Check sheet for the modelled part. Datum: model origin and axes. Units: mm. Face numbers are marked on the shaded views. A direction names the side the tool comes from. Coordinates: 2 decimals unless noted, no trailing zeros. Loops run counter-clockwise (first coordinate to the right, second up) from the corner with the lowest first, then second, coordinate; pieces in that order, holes last. Notation, with made-up numbers: M 16.5,-8 L 42.5,-8 A13 ccw 42.5,12 Z; hole C 14,50 d11. An arc over 180 degrees is marked long. Use CSV: the item, a comma, the result in double quotes. Start each with the question number.
(1) Section check B-B on y = 2. Record the cut outline in (x, z).
(2) Go/stop test with flat-tipped pins: pin 1 Ø1 at (x, z) = (-1, 1.5) entering from -Y; pin 2 Ø1.5 at (x, z) = (5.5, 1) entering from -Y; pin 3 Ø1.5 at (y, z) = (18.5, 2) entering from +X; pin 4 Ø1.5 at (x, z) = (-11.5, 1) entering from +Y. Record where each tip stops, or that it passes through.
(3) Scan lines: line 1 (X direction, y = -4, z = 1.05); line 2 (X direction, y = 18.5, z = 2.95); line 3 (Y direction, x = 12.25, z = 2.25). Record each from-to range of solid material in increasing order.
(4) Section check D-D on x = 0. Record the cut outline in (y, z), and give its area (3 significant figures).
(5) Section check A-A on z = 0.95. Record the cut outline in (x, y), and give its area (3 significant figures).
(6) Section check C-C on x = -7. Record the cut outline in (y, z), and give its area (3 significant figures).
(7) Draft check along X on the marked faces 4, 5, 6 and 7. Enter one of: pulls with the +X half, pulls with the -X half, needs draft (parallel to the pull), parting line crosses it, or undercut.
(8) Set-up check for the marked faces 1, 2 and 3: record each of +Z, -Z, +X, -X, +Y, -Y from which the full face is reachable in a straight line by a thin tool's end or side.
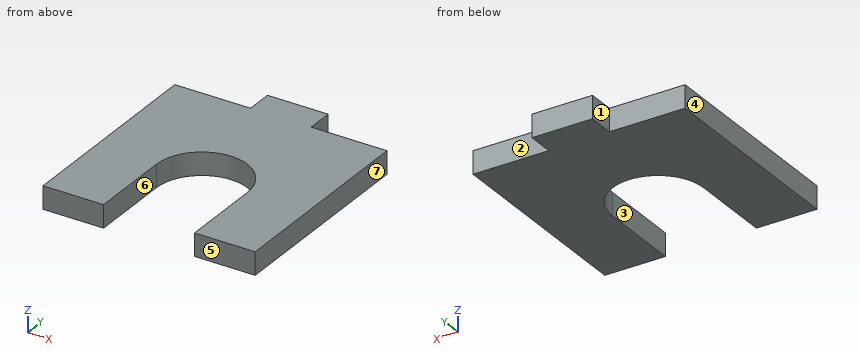
from build123d import *

# Parameters (mm, degrees)
RESSALTO_EXTRUS_O1_DEPTH = 3


with BuildPart() as part:
    # Esboço9 → Ressalto-extrusão1 (new body)
    with BuildSketch(Plane.XY):
        with BuildLine():
            Line((-14, -10.9375), (-6, -10.9375))
            Line((-6, -10.9375), (-6, 0))
            ThreePointArc((-6, 0), (0, 6), (6, 0))
            Line((6, 0), (6, -10.9375))
            Line((6, -10.9375), (14, -10.9375))
            Line((14, -10.9375), (14, 16.367680587))
            Line((14, 16.367680587), (4, 16.367680587))
            Line((4, 16.367680587), (4, 19.867680587))
            Line((4, 19.867680587), (-4, 19.867680587))
            Line((-4, 19.867680587), (-4, 16.367680587))
            Line((-4, 16.367680587), (-14, 16.367680587))
            Line((-14, 16.367680587), (-14, -10.9375))
        make_face()
    extrude(amount=RESSALTO_EXTRUS_O1_DEPTH)


solid = part.part
Outcome:
1,outline,"M -14,0 L -5.66,0 L -5.66,3 L -14,3 Z; M 5.66,0 L 14,0 L 14,3 L 5.66,3 Z"
2,pin 1,"stops at y = 5.81"
2,pin 2,"stops at y = -10.94"
2,pin 3,"stops at x = 4"
2,pin 4,"stops at y = 16.37"
3,line 1,"x = -14 to -6, 6 to 14"
3,line 2,"x = -4 to 4"
3,line 3,"y = -10.94 to 16.37"
4,outline,"M 6,0 L 19.87,0 L 19.87,3 L 6,3 Z"
4,area,"41.6 mm²"
5,outline,"M -14,-10.94 L -6,-10.94 L -6,0 A6 cw 6,0 L 6,-10.94 L 14,-10.94 L 14,16.37 L 4,16.37 L 4,19.87 L -4,19.87 L -4,16.37 L -14,16.37 Z"
5,area,"605 mm²"
6,outline,"M -10.94,0 L 16.37,0 L 16.37,3 L -10.94,3 Z"
6,area,"81.9 mm²"
7,face 4,"pulls with the -X half"
7,face 5,"needs draft"
7,face 6,"undercut"
7,face 7,"pulls with the +X half"
8,face 1,"+Z, -Z, -X, +Y"
8,face 2,"+Z, -Z, +X, +Y"
8,face 3,"+Z, -Z, -Y"
